Can you work these out from the model? Positions are in its coordinate system, mm. A direction names the side the tool comes from. Round coordinates to 2 decimals unless told otherwise and drop trailing zeros. Loops run counter-clockwise (first coordinate to the right, second up) from the corner with the lowest first, then second, coordinate; pieces in that order, holes last. Notation, with made-up numbers: (27, 64) -> (65, 64) arc R16 cw to (65, 93) -> close; hole circle Ø3 at (-27.75, 31). An arc over 180 degrees is marked (long way). Answer as a JSON object with one key per item and string values.
```python
from build123d import *

# Parameters (mm, degrees)
F0_W      = 25
F0_H      = 10
F0_W_2    = 10
F0_H_2    = 4.25
F1_DEPTH  = 2.5
F3_DEPTH  = 2.5
F4_DEPTH  = 18.5
F5_SIZE   = 4.2
F6_W      = 10
F6_H      = 4.25
F6_H_2    = 10
F6_H_3    = 10.75
F7_DEPTH  = 2.5
F8_DEPTH  = 20
F10_DEPTH = 60
F12_DEPTH = 10


with BuildPart() as f1:
    # F0 (on Top) → F1 (new body)
    with BuildSketch(Plane.XY):
        with Locations((-17.5, 0)):
            Rectangle(F0_W, F0_H)
        with Locations((0, 7.125)):
            Rectangle(F0_W_2, F0_H_2)
        Rectangle(F0_W_2, F0_H)
        with Locations((0, -7.125)):
            Rectangle(F0_W_2, F0_H_2)
        with Locations((17.5, 0)):
            Rectangle(F0_W, F0_H)
    extrude(amount=F1_DEPTH)

    # F2 (on face) → F3 (join)
    with BuildSketch(Plane.XZ.offset(9.25)):
        with BuildLine():
            Line((0, 0), (-5, 0))
            Line((-5, 0), (-5, -5))
            ThreePointArc((-5, -5), (-3.5355339059, -1.4644660941), (0, 0))
        make_face()
        with BuildLine():
            Line((5, 0), (0, 0))
            ThreePointArc((0, 0), (3.5355339059, -1.4644660941), (5, -5))
            Line((5, -5), (5, 0))
        make_face()
        with BuildLine():
            ThreePointArc((5, -5), (3.5355339059, -1.4644660941), (0, 0))
            ThreePointArc((0, 0), (-3.5355339059, -1.4644660941), (-5, -5))
            Line((-5, -5), (-2.5, -5))
            ThreePointArc((-2.5, -5), (0, -2.5), (2.5, -5))
            Line((2.5, -5), (5, -5))
        make_face()
        with BuildLine():
            Line((-2.5, -5), (-5, -5))
            ThreePointArc((-5, -5), (0, -10), (5, -5))
            Line((5, -5), (2.5, -5))
            ThreePointArc((2.5, -5), (0, -7.5), (-2.5, -5))
        make_face()
        with BuildLine():
            Line((2.5, -5), (-2.5, -5))
            ThreePointArc((-2.5, -5), (0, -7.5), (2.5, -5))
        make_face()
        with BuildLine():
            ThreePointArc((2.5, -5), (0, -2.5), (-2.5, -5))
            Line((-2.5, -5), (2.5, -5))
        make_face()
        Polygon((-5, 2.5), (-5, 0), (0, 0), (5, 0), (5, 2.5), align=None)
    extrude(amount=F3_DEPTH)

    # F2 (on face) → F4 (join)
    with BuildSketch(Plane.XZ.offset(9.25)):
        with BuildLine():
            ThreePointArc((5, -5), (3.5355339059, -1.4644660941), (0, 0))
            ThreePointArc((0, 0), (-3.5355339059, -1.4644660941), (-5, -5))
            Line((-5, -5), (-2.5, -5))
            ThreePointArc((-2.5, -5), (0, -2.5), (2.5, -5))
            Line((2.5, -5), (5, -5))
        make_face()
        with BuildLine():
            Line((-2.5, -5), (-5, -5))
            ThreePointArc((-5, -5), (0, -10), (5, -5))
            Line((5, -5), (2.5, -5))
            ThreePointArc((2.5, -5), (0, -7.5), (-2.5, -5))
        make_face()
        with BuildLine():
            Line((0, 0), (-5, 0))
            Line((-5, 0), (-5, -5))
            ThreePointArc((-5, -5), (-3.5355339059, -1.4644660941), (0, 0))
        make_face()
        with BuildLine():
            Line((5, 0), (0, 0))
            ThreePointArc((0, 0), (3.5355339059, -1.4644660941), (5, -5))
            Line((5, -5), (5, 0))
        make_face()
    extrude(amount=-F4_DEPTH)

    # F5
    f5_edges = [f1.edges().sort_by_distance(p)[0] for p in [
        (-5, 5, 1.25),
        (-5, -5, 1.25),
        (5, 5, 1.25),
        (5, -5, 1.25),
    ]]
    chamfer(f5_edges, length=F5_SIZE)

    # F6 (on face) → F7 (join)
    with BuildSketch(Plane.XY.offset(2.5)):
        with Locations((-25, 7.125)):
            Rectangle(F6_W, F6_H)
        with Locations((-25, 0)):
            Rectangle(F6_W, F6_H_2)
        with Locations((-25, -10.375)):
            Rectangle(F6_W, F6_H_3)
        with Locations((25, 7.125)):
            Rectangle(F6_W, F6_H)
        with Locations((25, 0)):
            Rectangle(F6_W, F6_H_2)
        with Locations((25, -10.375)):
            Rectangle(F6_W, F6_H_3)
    extrude(amount=-F7_DEPTH)

    # F6 (on face) → F8 (join)
    with BuildSketch(Plane.XY.offset(2.5)):
        with Locations((-25, 7.125)):
            Rectangle(F6_W, F6_H)
        with Locations((-25, 0)):
            Rectangle(F6_W, F6_H_2)
        with Locations((-25, -10.375)):
            Rectangle(F6_W, F6_H_3)
        with Locations((25, -10.375)):
            Rectangle(F6_W, F6_H_3)
        with Locations((25, 0)):
            Rectangle(F6_W, F6_H_2)
        with Locations((25, 7.125)):
            Rectangle(F6_W, F6_H)
    extrude(amount=F8_DEPTH)

    # F9 (on face) → F10 (cut)
    with BuildSketch(Plane(origin=(-30, 0, 0), x_dir=(0, -1, 0), z_dir=(-1, 0, 0))):
        with BuildLine():
            ThreePointArc((8.403882032, 2.5), (12.855823048, 6.644176952), (14.5, 12.5))
            ThreePointArc((14.5, 12.5), (12.855823048, 18.355823048), (8.403882032, 22.5))
            Line((8.403882032, 22.5), (3.25, 22.5))
            Line((3.25, 22.5), (-1.903882032, 22.5))
            ThreePointArc((-1.903882032, 22.5), (-6.355823048, 18.355823048), (-8, 12.5))
            ThreePointArc((-8, 12.5), (-6.355823048, 6.644176952), (-1.903882032, 2.5))
            Line((-1.903882032, 2.5), (8.403882032, 2.5))
        make_face()
        with BuildLine():
            ThreePointArc((8.403882032, 22.5), (12.855823048, 18.355823048), (14.5, 12.5))
            Line((14.5, 12.5), (14.5, 22.5))
            Line((14.5, 22.5), (8.403882032, 22.5))
        make_face()
        with BuildLine():
            ThreePointArc((-8, 12.5), (-6.355823048, 18.355823048), (-1.903882032, 22.5))
            Line((-1.903882032, 22.5), (-8, 22.5))
            Line((-8, 22.5), (-8, 12.5))
        make_face()
    extrude(amount=-F10_DEPTH, mode=Mode.SUBTRACT)

    # F11 (on face) → F12 (cut)
    with BuildSketch(Plane.XZ.offset(15.75)):
        with BuildLine():
            Line((-25, 15), (-25, 16.3))
            ThreePointArc((-25, 16.3), (-25.9192388155, 14.0807611845), (-23.7, 15))
            Line((-23.7, 15), (-25, 15))
        make_face()
        with BuildLine():
            ThreePointArc((-23.7, 15), (-24.0807611845, 15.9192388155), (-25, 16.3))
            Line((-25, 16.3), (-25, 15))
            Line((-25, 15), (-23.7, 15))
        make_face()
        with BuildLine():
            ThreePointArc((26.3, 15), (25, 16.3), (23.7, 15))
            ThreePointArc((23.7, 15), (25, 13.7), (26.3, 15))
        make_face()
    extrude(amount=-F12_DEPTH, mode=Mode.SUBTRACT)


solid = f1.part
```
Q1. We'd pull the mould along Z, two halves only. Please class faces 5 (the flat face through (15, 5, 1)), 6 (the cylindrical face through (-0.33, -0.13, -7.48)), 7 (the flat face through (-25, -15, 22.5)): pulls with the +Z half, pulls with the -Z half, needs draft (parallel to the pull), parting line crosses it, or undercut.
Determined:
{"face 5": "needs draft", "face 6": "undercut", "face 7": "pulls with the +Z half"}
Q2. I want a section at D-D, the plane x = -12. Write out the boundary of the cut face in (y, z), then the cut area to 3 significant figures.
Determined:
{"outline": "(-5, 0) -> (5, 0) -> (5, 2.5) -> (-5, 2.5) -> close", "area": "25.0 mm²"}
Q3. I want a section at B-B, the plane y = -2. Write out the boundary of the cut face in (x, z), then the cut area to 3 significant figures.
Determined:
{"outline": "(-30, 0) -> (-5, 0) -> (-5, -5) arc R5 ccw to (5, -5) -> (5, 0) -> (30, 0) -> (30, 2.5) -> (-30, 2.5) -> close; hole circle Ø5 at (0, -5)", "area": "220 mm²"}
Q4. I'm going to push flat-ended pins straight in: pin 1 (7.5 mm diameter, centred on x = 22, y = -4.5, fed in from -Z); pin 2 (2 mm diameter, centred on x = 16, z = 2, fed in from +Y); pin 3 (3 mm diameter, centred on x = -1.5, z = -1.5, fed in from -Y). Where does each tip first touch, or does it pass through?
Determined:
{"pin 1": "z = 0", "pin 2": "y = 5", "pin 3": "y = -11.75"}
Q5. I want a section at A-A, the plane x = 25. Write out the boundary of the cut face in (y, z).
Determined:
{"outline": "(-15.75, 0) -> (9.25, 0) -> (9.25, 22.5) -> (8, 22.5) -> (8, 12.5) arc R11.25 cw to (1.9, 2.5) -> (-8.4, 2.5) arc R11.25 cw to (-14.5, 12.5) -> (-14.5, 13.7) -> (-15.75, 13.7) -> close; (-15.75, 16.3) -> (-14.5, 16.3) -> (-14.5, 22.5) -> (-15.75, 22.5) -> close"}
Q6. I want a section at C-C, the plane z = 9.5. Write out the boundary of the cut face in (x, y).
Determined:
{"outline": "(-30, -15.75) -> (-20, -15.75) -> (-20, -14.09) -> (-30, -14.09) -> close; (-30, 7.59) -> (-20, 7.59) -> (-20, 9.25) -> (-30, 9.25) -> close; (20, -15.75) -> (30, -15.75) -> (30, -14.09) -> (20, -14.09) -> close; (20, 7.59) -> (30, 7.59) -> (30, 9.25) -> (20, 9.25) -> close"}
Q7. On a 3-axis mill with a long thin cutter (end or side, diameter ignored), from which of +Z, -Z, +X, -X, +Y, -Y can I reach the whole of each face in a straight line? I mean faces 1 (the flat face through (-20, -13, 6)), 2 (the cylindrical face through (24.93, 6.4, 6.72)), 3 (the flat face through (0, -9.25, -5)), 4 (the flat face through (0, -1, 2.5)). Say none if no direction works.
Determined:
{"face 1": "+Z, -Z, -Y", "face 2": "+Z, +X, -X", "face 3": "+Y", "face 4": "+Z"}
Q8. If I drill on L1, parallel to X at y = -15, z = 15; L2, parallel to Y at x = 21, z = 14; L3, parallel to Z at x = 25, y = -15.3, over which ranges is the centre line in solid material (lowest first)? Write a range as [from, to].
Determined:
{"L1": "[-30, -26.3], [-23.7, -20], [20, 23.7], [26.3, 30]", "L2": "[-15.75, -14.5], [8, 9.25]", "L3": "[0, 13.7], [16.3, 22.5]"}
